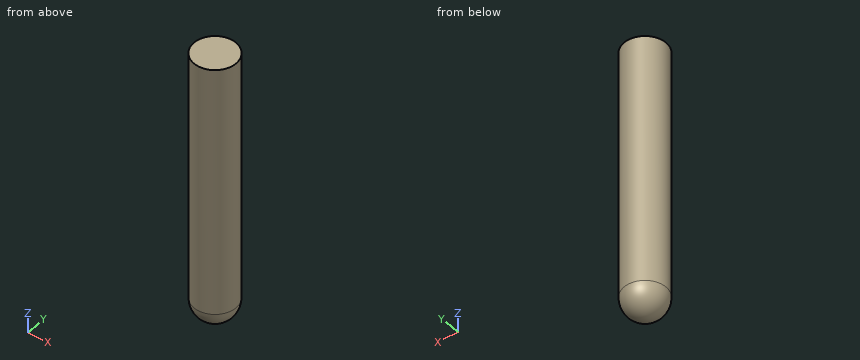
from build123d import *

# Parameters (mm, degrees)
CYLINDER001_R     = 5
CYLINDER001_DEPTH = 60


with BuildPart() as cylinder001:
    # Cylinder001 → Cylinder001 (new body)
    with BuildSketch(Plane.XY):
        Circle(CYLINDER001_R)
    extrude(amount=CYLINDER001_DEPTH)


with BuildPart() as fusion001:
    # Sphere → Sphere (revolve)
    with BuildSketch(Plane.XZ):
        with BuildLine():
            ThreePointArc((0, -5), (5, 0), (0, 5))
            Line((0, 5), (0, -5))
        make_face()
    revolve(axis=Axis((0, 0, 0), (0, 0, 1)))

    # Fusion001: union Cylinder001
    add(cylinder001.part)


with BuildPart() as fusion001_1:
    # Fusion001 placement: moved
    add(fusion001.part.moved(Location((0, 0, 30))))


solid = fusion001_1.part
Here's how the part is built. I have some questions about the finished solid (model axes, mm). Round coordinates to 2 decimals unless told otherwise and drop trailing zeros. Loops run counter-clockwise (first coordinate to the right, second up) from the corner with the lowest first, then second, coordinate; pieces in that order, holes last. Notation, with made-up numbers: (-36, 27.25) - (8, 27.25) arc R11 cw to (8, 43.25) - close; hole circle Ø9 at (-15.5, 84.5). An arc over 180 degrees is marked (long way). One line per question, with ' | ' between items. Start each with the question number.
Q1. I want a section at A-A (y = 0). Write out the boundary of the cut face in (x, z).
Q2. Will these pins go through, and if not, where does the flat tip stop? pin 1 (1.5 mm diameter, centred on y = 1, z = 72, fed in from +X); pin 2 (1.5 mm diameter, centred on y = 2.5, z = 62.5, fed in from -X); pin 3 (1 mm diameter, centred on x = -0.5, y = 3.5, fed in from -Z).
Q3. Please list where these lines run through material, in increasing order: line 1 (Y direction, x = 0.25, z = 50); line 2 (Z direction, x = 1.75, y = 3.5); line 3 (Z direction, x = -3.75, y = 1.5). Write a range as [from, to].
Q4. I want a section at C-C (z = 33.5). Write out the boundary of the cut face in (x, y), then the cut area to 3 significant figures.
Response values:
1) outline: (-5, 30) arc R5 ccw to (5, 30) - (5, 90) - (-5, 90) - close
2) pin 1: stops at x = 4.99 | pin 2: stops at x = -4.68 | pin 3: stops at z = 26.03
3) line 1: y = [-4.99, 4.99] | line 2: z = [26.89, 90] | line 3: z = [27.05, 90]
4) outline: circle Ø10 at (0, 0) | area: 78.5 mm²
